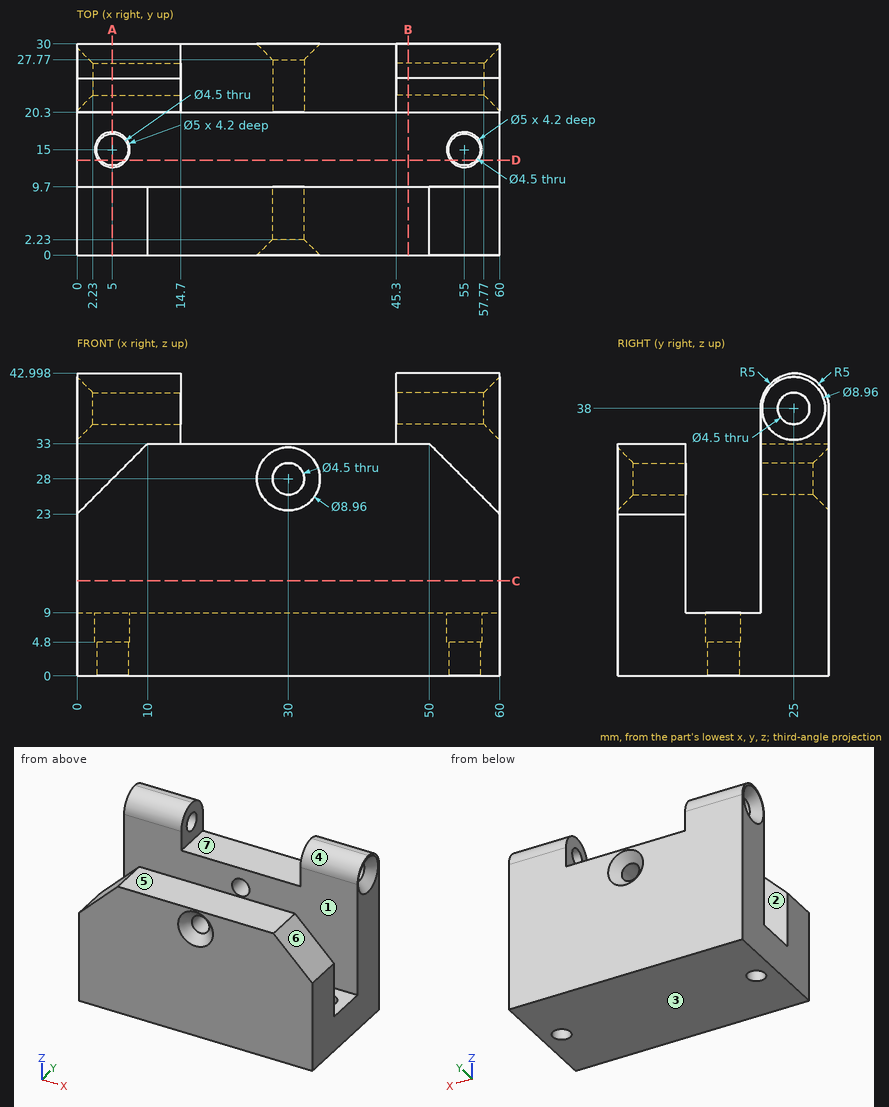
The drawing under review shows one solid part. Ordinate dimensions are in mm from its lowest x, y, z. A direction names the side the tool comes from. Give positions to 0.01 mm unless a question says otherwise; leave off trailing zeros. Loops run counter-clockwise (first coordinate to the right, second up) from the corner with the lowest first, then second, coordinate; pieces in that order, holes last. Notation, with made-up numbers: M 6,9 L 60,9 A16 cw 60,29 Z; hole C -0.5,54 d6. An arc over 180 degrees is marked long. One line per question, with ' | ' between items. Start each with the question number.
1. For the marked faces 5, 6 and 7, list the 3-axis set-ups (+Z, -Z, +X, -X, +Y, -Y) from which the entire face can be reached by the end or side of a thin tool; tool diameter is ignored.
2. Add section D-D (y = 13.5). Write out the cut boundary in (x, z), plus the area to 3 significant figures.
3. Insertion check: P1, Ø6.5, axis at x = 55, y = 15, coming from the +Z side; P2, Ø6, axis at x = 30, z = 28, coming from the +Y side; P3, Ø6, axis at x = 16.5, y = 5, coming from the +Z side. Each pin has a flat end and moves straight along its axis. Give the tip position at first contact, or say it passes through.
4. To check wall thickness, follow L1, parallel to X at y = 26, z = 28; L2, parallel to Y at x = 47.5, z = 26.5; L3, parallel to Y at x = 55, z = 2.4. State the ranges of each line that lie inside material, in increasing order.
5. The part is to be moulded in two halves that separate along Y. For the marked faces 1, 2, 3 and 4, say which applies: released by +Y, released by -Y, zero draft, split by the parting line, or undercut.
6. Add section B-B (x = 47). Write out the cut boundary in (y, z), plus the area to 3 significant figures.
7. Add section C-C (z = 13.5). Write out the cut boundary in (x, y), plus the area to 3 significant figures.
8. Add section A-A (x = 5). Write out the cut boundary in (y, z), plus the area to 3 significant figures.
Worked out:
1) face 5: +Z, +X, -X, -Y | face 6: +Z, +X, -Y | face 7: +Z, +Y, -Y
2) outline: M 0,0 L 3.32,0 L 3.32,4.8 L 3,4.8 L 3,9 L 0,9 Z; M 6.68,0 L 53.32,0 L 53.32,4.8 L 53,4.8 L 53,9 L 7,9 L 7,4.8 L 6.68,4.8 Z; M 56.68,0 L 60,0 L 60,9 L 57,9 L 57,4.8 L 56.68,4.8 Z | area: 474 mm²
3) P1: stops at z = 9 | P2: stops at y = 28.52 | P3: stops at z = 33
4) L1: x = 0 to 27.75, 32.25 to 60 | L2: y = 0 to 9.7, 20.3 to 30 | L3: y = 0 to 12.75, 17.25 to 30
5) face 1: undercut | face 2: undercut | face 3: zero draft | face 4: released by -Y
6) outline: M 0,0 L 30,0 L 30,38 A5 ccw 25.15,43 A5 ccw 20.3,38 L 20.3,9 L 9.7,9 L 9.7,33 L 0,33 Z; hole C 25,38 d4.5 | area: 806 mm²
7) outline: M 0,0 L 60,0 L 60,9.7 L 0,9.7 Z; M 0,20.3 L 60,20.3 L 60,30 L 0,30 Z | area: 1,160 mm²
8) outline: M 0,0 L 12.75,0 L 12.75,4.8 L 12.5,4.8 L 12.5,9 L 9.7,9 L 9.7,28 L 0,28 Z; M 17.25,0 L 30,0 L 30,38 A5 ccw 25.15,43 A5 ccw 20.3,38 L 20.3,9 L 17.5,9 L 17.5,4.8 L 17.25,4.8 Z; hole C 25,38 d4.5 | area: 715 mm²
